Geometry check sheet. Reference: the model listing, model coordinates, mm. A direction names the side the tool comes from. Coordinates: 2 decimals unless noted, no trailing zeros. Order: outer loops, then holes, each group sorted by start corner. A loop starts at its lowest first (then second) coordinate and runs counter-clockwise, first axis right, second up. Notation, with made-up numbers: (-27, 34) - (1, 34) arc R19 ccw to (1, 46) - close; hole circle Ø3 at (-21.75, 47.5). An arc over 180 degrees is marked (long way). Use CSV: the item, a comma, the result in double quotes. Start each with the question number.
1) Depth check by flat-ended pin: P1, Ø3.5, axis at x = -45.83, z = 30.48, coming from the -Y side; P2, Ø4.5, axis at x = -45.83, z = -30.48, coming from the +Y side; P3, Ø1.1, axis at x = 13, y = 2.5, coming from the +Z side; P4, Ø1.8, axis at x = 45.83, z = -30.48, coming from the +Y side. Enter the tip coordinate at first touch or a pass-through.
2) Sectioned sample at A-A, the plane x = 34.5. Record the cut outline in (y, z).
3) Sectioned sample at B-B, the plane y = -1.25. Record the cut outline in (x, z).
4) Thickness scan on probe 1 along X at (y, z) = (0.25, -24); probe 2 along X at (y, z) = (1.25, 1.27); probe 3 along Z at (x, y) = (-25, 0.5). Record the ranges inside material, lowest first. Write a range as [from, to].
5) Draft check along Z on faces 1 (the cylindrical face through (44.76, 0.8, 29.49)), 2 (the cylindrical face through (-45.89, 0.8, 33.02)), 3 (the flat face through (-43, 1.626, 0)). Enter one of: released by +Z, released by -Z, zero draft, split by the parting line, or undercut.
6) Tool access check on faces 4 (the flat face through (1, 0, -28.067)), 5 (the flat face through (-1, 3, 27.813)), 6 (the flat face through (37.452, -1, 0)), 7 (the flat face through (-1, 3, -27.813)), 8 (the flat face through (-41, 0, 0)). Record the directions out of +Z, -Z, +X, -X, +Y, -Y that give a thin tool (end or side, any length) a straight path to the whole face; none if there is none.
from build123d import *

# Parameters (mm, degrees)
SKETCH1_R           = 1.4605
SKETCH1_R_2         = 0.4318
SKETCH1_W           = 85.0392
SKETCH1_H           = 55.626
BOSS_EXTRUDE1_DEPTH = 1.6256
SKETCH1_2_W         = 85.0392
SKETCH1_2_H         = 55.626
BOSS_EXTRUDE2_DEPTH = 5.334
SKETCH2_W           = 71.8566
SKETCH2_H           = 56.134
BOSS_EXTRUDE3_DEPTH = 2.54


with BuildPart() as part:
    # Sketch1 → Boss-Extrude1 (new body)
    with BuildSketch(Plane(origin=(0, 0, 0), x_dir=(1, 0, 0), z_dir=(0, 1, 0))):
        with BuildLine():
            Line((43.2943, 28.067), (-43.2943, 28.067))
            Line((-43.2943, 28.067), (-43.2943, 30.48))
            ThreePointArc((-43.2943, 30.48), (-45.8343, 33.02), (-48.3743, 30.48))
            Line((-48.3743, 30.48), (-48.3743, -30.48))
            ThreePointArc((-48.3743, -30.48), (-45.8343, -33.02), (-43.2943, -30.48))
            Line((-43.2943, -30.48), (-43.2943, -28.067))
            Line((-43.2943, -28.067), (43.2943, -28.067))
            Line((43.2943, -28.067), (43.2943, -30.48))
            ThreePointArc((43.2943, -30.48), (45.8343, -33.02), (48.3743, -30.48))
            Line((48.3743, -30.48), (48.3743, 30.48))
            ThreePointArc((48.3743, 30.48), (45.8343, 33.02), (43.2943, 30.48))
            Line((43.2943, 30.48), (43.2943, 28.067))
        make_face()
        with Locations((-45.8343, 30.48)):
            Circle(SKETCH1_R, mode=Mode.SUBTRACT)
        with Locations((-45.8343, -30.48)):
            Circle(SKETCH1_R, mode=Mode.SUBTRACT)
        with Locations((45.8343, -30.48)):
            Circle(SKETCH1_R, mode=Mode.SUBTRACT)
        with Locations((45.8343, 30.48)):
            Circle(SKETCH1_R, mode=Mode.SUBTRACT)
        with Locations((-45.8343, 24.13)):
            Circle(SKETCH1_R_2, mode=Mode.SUBTRACT)
        with Locations((-45.8343, 21.59)):
            Circle(SKETCH1_R_2, mode=Mode.SUBTRACT)
        with Locations((-45.8343, 19.05)):
            Circle(SKETCH1_R_2, mode=Mode.SUBTRACT)
        with Locations((-45.8343, 16.51)):
            Circle(SKETCH1_R_2, mode=Mode.SUBTRACT)
        with Locations((-45.8343, 13.97)):
            Circle(SKETCH1_R_2, mode=Mode.SUBTRACT)
        with Locations((-45.8343, 11.43)):
            Circle(SKETCH1_R_2, mode=Mode.SUBTRACT)
        with Locations((-45.8343, 8.89)):
            Circle(SKETCH1_R_2, mode=Mode.SUBTRACT)
        with Locations((-45.8343, 6.35)):
            Circle(SKETCH1_R_2, mode=Mode.SUBTRACT)
        with Locations((-45.8343, 3.81)):
            Circle(SKETCH1_R_2, mode=Mode.SUBTRACT)
        with Locations((-45.8343, 1.27)):
            Circle(SKETCH1_R_2, mode=Mode.SUBTRACT)
        with Locations((-45.8343, -1.27)):
            Circle(SKETCH1_R_2, mode=Mode.SUBTRACT)
        with Locations((-45.8343, -3.81)):
            Circle(SKETCH1_R_2, mode=Mode.SUBTRACT)
        with Locations((-45.8343, -6.35)):
            Circle(SKETCH1_R_2, mode=Mode.SUBTRACT)
        with Locations((-45.8343, -8.89)):
            Circle(SKETCH1_R_2, mode=Mode.SUBTRACT)
        with Locations((-45.8343, -11.43)):
            Circle(SKETCH1_R_2, mode=Mode.SUBTRACT)
        with Locations((-45.8343, -13.97)):
            Circle(SKETCH1_R_2, mode=Mode.SUBTRACT)
        with Locations((-45.8343, -16.51)):
            Circle(SKETCH1_R_2, mode=Mode.SUBTRACT)
        with Locations((-45.8343, -19.05)):
            Circle(SKETCH1_R_2, mode=Mode.SUBTRACT)
        with Locations((-45.8343, -21.59)):
            Circle(SKETCH1_R_2, mode=Mode.SUBTRACT)
        with Locations((-45.8343, -24.13)):
            Circle(SKETCH1_R_2, mode=Mode.SUBTRACT)
        with Locations((45.8343, -24.13)):
            Circle(SKETCH1_R_2, mode=Mode.SUBTRACT)
        with Locations((45.8343, -21.59)):
            Circle(SKETCH1_R_2, mode=Mode.SUBTRACT)
        with Locations((45.8343, -19.05)):
            Circle(SKETCH1_R_2, mode=Mode.SUBTRACT)
        with Locations((45.8343, -16.51)):
            Circle(SKETCH1_R_2, mode=Mode.SUBTRACT)
        with Locations((45.8343, -13.97)):
            Circle(SKETCH1_R_2, mode=Mode.SUBTRACT)
        with Locations((45.8343, -11.43)):
            Circle(SKETCH1_R_2, mode=Mode.SUBTRACT)
        with Locations((45.8343, -8.89)):
            Circle(SKETCH1_R_2, mode=Mode.SUBTRACT)
        with Locations((45.8343, -6.35)):
            Circle(SKETCH1_R_2, mode=Mode.SUBTRACT)
        with Locations((45.8343, -3.81)):
            Circle(SKETCH1_R_2, mode=Mode.SUBTRACT)
        with Locations((45.8343, -1.27)):
            Circle(SKETCH1_R_2, mode=Mode.SUBTRACT)
        with Locations((45.8343, 1.27)):
            Circle(SKETCH1_R_2, mode=Mode.SUBTRACT)
        with Locations((45.8343, 3.81)):
            Circle(SKETCH1_R_2, mode=Mode.SUBTRACT)
        with Locations((45.8343, 6.35)):
            Circle(SKETCH1_R_2, mode=Mode.SUBTRACT)
        with Locations((45.8343, 8.89)):
            Circle(SKETCH1_R_2, mode=Mode.SUBTRACT)
        with Locations((45.8343, 11.43)):
            Circle(SKETCH1_R_2, mode=Mode.SUBTRACT)
        with Locations((45.8343, 13.97)):
            Circle(SKETCH1_R_2, mode=Mode.SUBTRACT)
        with Locations((45.8343, 16.51)):
            Circle(SKETCH1_R_2, mode=Mode.SUBTRACT)
        with Locations((45.8343, 19.05)):
            Circle(SKETCH1_R_2, mode=Mode.SUBTRACT)
        with Locations((45.8343, 21.59)):
            Circle(SKETCH1_R_2, mode=Mode.SUBTRACT)
        with Locations((45.8343, 24.13)):
            Circle(SKETCH1_R_2, mode=Mode.SUBTRACT)
        Rectangle(SKETCH1_W, SKETCH1_H, mode=Mode.SUBTRACT)
    extrude(amount=BOSS_EXTRUDE1_DEPTH)

    # Sketch1<2> → Boss-Extrude2 (add)
    with BuildSketch(Plane(origin=(0, 0, 0), x_dir=(1, 0, 0), z_dir=(0, 1, 0))):
        Rectangle(SKETCH1_2_W, SKETCH1_2_H)
    extrude(amount=BOSS_EXTRUDE2_DEPTH)

    # Sketch2 → Boss-Extrude3 (add)
    with BuildSketch(Plane.XZ):
        with Locations((1.524, 0)):
            Rectangle(SKETCH2_W, SKETCH2_H)
    extrude(amount=BOSS_EXTRUDE3_DEPTH)


solid = part.part
Evaluation:
1,P1,"y = 0"
1,P2,"y = 1.63"
1,P3,"z = 27.81"
1,P4,"through"
2,outline,"(-2.54, -28.07) - (1.63, -28.07) - (1.63, -27.81) - (5.33, -27.81) - (5.33, 27.81) - (1.63, 27.81) - (1.63, 28.07) - (-2.54, 28.07) - close"
3,outline,"(-34.4, -28.07) - (37.45, -28.07) - (37.45, 28.07) - (-34.4, 28.07) - close"
4,probe 1,"[-48.37, -46.25], [-45.42, 45.42], [46.25, 48.37]"
4,probe 2,"[-48.37, -46.27], [-45.4, 45.4], [46.27, 48.37]"
4,probe 3,"[-28.07, 28.07]"
5,face 1,"undercut"
5,face 2,"released by +Z"
5,face 3,"zero draft"
6,face 4,"-Z, +Y, -Y"
6,face 5,"+Z, +X, -X, +Y"
6,face 6,"+Z, -Z, +X, -Y"
6,face 7,"-Z, +X, -X, +Y"
6,face 8,"+Z, -Z, -X, -Y"
